from build123d import *

# Parameters (mm, degrees)
F0_R          = 14
F0_R_2        = 1.4
F0_R_3        = 5
F1_DEPTH      = 1.7
F2_SIZE       = 0.2
F3_R          = 5
F4_DEPTH      = 4
F5_R          = 2.5
F6_DEPTH      = 1
F6_DEPTH_BACK = 4.001


with BuildPart() as f1:
    # F0 (on Front) → F1 (new body)
    with BuildSketch(Plane.XZ):
        Circle(F0_R)
        with Locations((-8, 0)):
            Circle(F0_R_2, mode=Mode.SUBTRACT)
        Circle(F0_R_3, mode=Mode.SUBTRACT)
        with Locations((8, 0)):
            Circle(F0_R_2, mode=Mode.SUBTRACT)
    extrude(amount=-F1_DEPTH)

    # F2
    f2_edges = [f1.edges().sort_by_distance(p)[0] for p in [
        (-14, 1.7, 0),
        (-14, 0, 0),
    ]]
    chamfer(f2_edges, length=F2_SIZE)

    # F3 (on face) → F4 (join)
    with BuildSketch(Plane.XZ):
        with BuildLine():
            ThreePointArc((-8.66265625, 1.2332423502), (-6.6, 0), (-8.66265625, -1.2332423502))
            ThreePointArc((-8.66265625, -1.2332423502), (0, -8.75), (8.66265625, -1.2332423502))
            ThreePointArc((8.66265625, -1.2332423502), (6.6, 0), (8.66265625, 1.2332423502))
            ThreePointArc((8.66265625, 1.2332423502), (0, 8.75), (-8.66265625, 1.2332423502))
        make_face()
        Circle(F3_R, mode=Mode.SUBTRACT)
    extrude(amount=F4_DEPTH)

    # F5 (on face) → F6 (cut, two sides)
    with BuildSketch(Plane.XZ) as f6_sk:
        with Locations((-8, 0)):
            Circle(F5_R)
        with Locations((8, 0)):
            Circle(F5_R)
    extrude(amount=-F6_DEPTH, mode=Mode.SUBTRACT)
    extrude(f6_sk.sketch, amount=F6_DEPTH_BACK, mode=Mode.SUBTRACT)


solid = f1.part
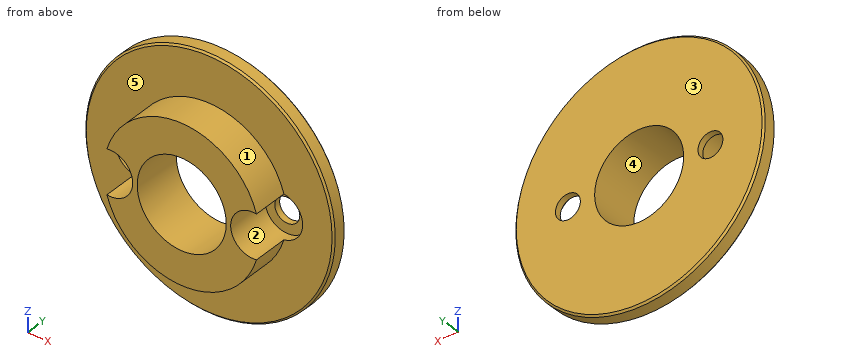
Geometry check sheet. Reference: the model listing, model coordinates, mm. Face numbers are marked on the shaded views. A direction names the side the tool comes from. Give positions to 0.01 mm unless a question says otherwise; leave off trailing zeros. Loops run counter-clockwise (first coordinate to the right, second up) from the corner with the lowest first, then second, coordinate; pieces in that order, holes last. Notation, with made-up numbers: M 80,30.25 L 137,30.25 A20 ccw 137,55.25 Z; hole C 80,-34 d4. An arc over 180 degrees is marked long. Answer as a JSON object with one key per item and string values. Group by question number.
Item 1: Gauge pin test, flat ends, axial feed: pin 1 (2 mm diameter, centred on x = -8, z = 0, fed in from -Y); pin 2 (3 mm diameter, centred on x = -5, z = -10, fed in from -Y); pin 3 (1.5 mm diameter, centred on x = -6.5, y = -2, fed in from -Z); pin 4 (1.5 mm diameter, centred on y = 1, z = -1, fed in from -X). Record the tip position at first contact, or that the pin passes through.
Item 2: Sectioned sample at A-A on x = 0. Record the boundary of the cut face in (y, z).
Item 3: Mould release check, pull along Z, two halves, no side actions. Record for the marked faces 1, 2 and 3: pulls with the +Z half, pulls with the -Z half, needs draft (parallel to the pull), parting line crosses it, or undercut.
Item 4: Sectioned sample at C-C on y = -3.5. Record the boundary of the cut face in (x, z), plus the area to 3 significant figures.
Item 5: Access from +Z, -Z, +X, -X, +Y, -Y to the whole of each face (thin tool, end or side, straight path). Record for the marked faces 4 and 5.
Item 6: Material ranges on L1, parallel to X at y = -2.05, z = 5.75; L2, parallel to Z at x = 6.25, y = 0.8; L3, parallel to X at y = 0.95, z = -3.5, recorded low to high.
Item 7: Sectioned sample at B-B on z = 0. Record the boundary of the cut face in (x, y).
Findings below:
{
 "1": {"pin 1": "through", "pin 2": "y = 0", "pin 3": "z = -6.6", "pin 4": "x = -14"},
 "2": {"outline": "M -4,-8.75 L 0,-8.75 L 0,-13.8 L 0.2,-14 L 1.5,-14 L 1.7,-13.8 L 1.7,-5 L -4,-5 Z; M -4,5 L 1.7,5 L 1.7,13.8 L 1.5,14 L 0.2,14 L 0,13.8 L 0,8.75 L -4,8.75 Z"},
 "3": {"face 1": "pulls with the +Z half", "face 2": "undercut", "face 3": "needs draft"},
 "4": {"outline": "M -8.39,-2.47 A8.75 ccw 8.39,-2.47 A2.5 cw long 8.39,2.47 A8.75 ccw -8.39,2.47 A2.5 cw long Z; hole C 0,0 d10", "area": "136 mm2"},
 "5": {"face 4": "+Y, -Y", "face 5": "-Y"},
 "6": {"L1": "-6.6 to 6.6", "L2": "-12.53 to -1.79, 1.79 to 12.53", "L3": "-13.56 to -3.57, 3.57 to 13.56"},
 "7": {"outline": "M -14,0.2 L -13.8,0 L -10.5,0 L -10.5,1 L -9.4,1 L -9.4,1.7 L -13.8,1.7 L -14,1.5 Z; M -6.6,1 L -5.5,1 L -5.5,-4 L -5,-4 L -5,1.7 L -6.6,1.7 Z; M 5,-4 L 5.5,-4 L 5.5,1 L 6.6,1 L 6.6,1.7 L 5,1.7 Z; M 9.4,1 L 10.5,1 L 10.5,0 L 13.8,0 L 14,0.2 L 14,1.5 L 13.8,1.7 L 9.4,1.7 Z"}
}
